Here's how the part is built. I have some questions about the finished solid (model axes, mm). Round coordinates to 2 decimals unless told otherwise and drop trailing zeros. Order: outer loops, then holes, each group sorted by start corner. A loop starts at its lowest first (then second) coordinate and runs counter-clockwise, first axis right, second up. Notation, with made-up numbers: M -33,15.25 L 22,15.25 A32 ccw 22,44.25 Z; hole C -9.75,50 d4. An arc over 180 degrees is marked long. Write each question's results on one line, items separated by ' | '. Start each with the question number.
```python
from build123d import *

# Parameters (mm, degrees)
SKETCH1_W           = 45
SKETCH1_H           = 20
BOSS_EXTRUDE1_DEPTH = 4
SKETCH2_R           = 1.25
CUT_EXTRUDE1_DEPTH  = 25.944939367
FILLET2_R           = 10


with BuildPart() as part:
    # Sketch1 → Boss-Extrude1 (new body)
    with BuildSketch(Plane(origin=(0, 0, 0), x_dir=(1, 0, 0), z_dir=(0, 1, 0))):
        Rectangle(SKETCH1_W, SKETCH1_H)
    extrude(amount=BOSS_EXTRUDE1_DEPTH)

    # Sketch2 → Cut-Extrude1 (cut, through all)
    with BuildSketch(Plane(origin=(0, 4, 0), x_dir=(1, 0, 0), z_dir=(0, 1, 0))):
        with Locations(Location((18, 0, 0), (0, 0, 270))):
            Circle(SKETCH2_R)
        with Locations(Location((-10, 0, 0), (0, 0, 270))):
            Circle(SKETCH2_R)
        with Locations(Location((-18, 0, 0), (0, 0, 270))):
            Circle(SKETCH2_R)
        with BuildLine():
            ThreePointArc((4.583333333, -2.338743727), (15.9, 0), (4.583333333, 2.338743727))
            ThreePointArc((4.583333333, 2.338743727), (1.2, 0), (4.583333333, -2.338743727))
        make_face()
    extrude(amount=-CUT_EXTRUDE1_DEPTH, mode=Mode.SUBTRACT)

    # Fillet2
    fillet2_edges = [part.edges().sort_by_distance(p)[0] for p in [
        (-22.5, 2, -10),
        (22.5, 2, -10),
        (-22.5, 2, 10),
        (22.5, 2, 10),
    ]]
    fillet(fillet2_edges, radius=FILLET2_R - 0.0001)  # a hair under: the kernel refuses the full size


solid = part.part
```
(1) I want a section at B-B on z = -0.75. Write out the boundary of the cut face in (x, y).
(2) I want a section at C-C on x = 10. Write out the boundary of the cut face in (y, z).
(3) Please list where these lines run through material, in increasing order: line 1 (X direction, y = 3.15, z = 0); line 2 (X direction, y = 3.45, z = 0.75); line 3 (X direction, y = 1.35, z = -2).
(4) I want a section at D-D on y = 2.7. Give the number of separate pieces and of enclosed holes in the cut face, and give its area (3 significant figures).
(5) I want a section at A-A on x = 3.7. Write out the boundary of the cut face in (y, z), and give its area (3 significant figures).
(6) I'm going to push flat-ended pins straight in: pin 1 Ø2 at (x, z) = (-18, 0) entering from +Y; pin 2 Ø1 at (y, z) = (1.5, 3) entering from +X; pin 3 Ø1 at (x, y) = (-18, 1) entering from +Z. Where does each tip first touch, or does it pass through?
(7) If we mould it in two halves opening along X, with no side actions, what happens to faces 1 (the flat face through (0, 2, 10)), 2 (the cylindrical face through (-19.65, 2.03, -6.99)), 3 (the cylindrical face through (-8.76, 2.03, -0.16))? For each: pulls with the +X half, pulls with the -X half, needs draft (parallel to the pull), parting line crosses it, or undercut.
Solutions:
1) outline: M -22.47,0 L -19,0 L -19,4 L -22.47,4 Z; M -17,0 L -11,0 L -11,4 L -17,4 Z; M -9,0 L 1.32,0 L 1.32,4 L -9,4 Z; M 15.85,0 L 17,0 L 17,4 L 15.85,4 Z; M 19,0 L 22.47,0 L 22.47,4 L 19,4 Z
2) outline: M 0,-10 L 4,-10 L 4,-5.9 L 0,-5.9 Z; M 0,5.9 L 4,5.9 L 4,10 L 0,10 Z
3) line 1: -22.5 to -19.25, -16.75 to -11.25, -8.75 to 1.2, 15.9 to 16.75, 19.25 to 22.5 | line 2: -22.47 to -19, -17 to -11, -9 to 1.32, 15.85 to 17, 19 to 22.47 | line 3: -22.3 to 2.2, 15.55 to 22.3
4) separate pieces: 1 | enclosed holes: 4 | area: 677 mm^2
5) outline: M 0,-10 L 4,-10 L 4,-2.5 L 0,-2.5 Z; M 0,2.5 L 4,2.5 L 4,10 L 0,10 Z | area: 60.0 mm^2
6) pin 1: through | pin 2: x = 22.18 | pin 3: z = 8.66
7) face 1: needs draft | face 2: pulls with the -X half | face 3: undercut
